Input: part model. Units: mm. Frame: model coordinates. Face numbers are marked on the shaded views. Give positions to 0.01 mm unless a question says otherwise; leave off trailing zeros. Write each loop counter-clockwise with the first axis right and the second up, starting at its lowest first coordinate (ties: lowest second). Pieces come first, ordered by that corner, then holes. Notation, with made-up numbers: (-37.75, 8.5) -> (-14.75, 8.5) arc R24 ccw to (-14.75, 31.5) -> close; hole circle Ø10 at (69.5, 38). An arc over 180 degrees is marked (long way). Return JSON: item names as keys, results as strings. Group by question number.
Item 1: Section A-A, the plane z = 0.5. Return loops of the section in (x, y), then the cut area to 3 significant figures.
Item 2: Pin query (flat end, axial travel): P1, Ø0.5, axis at y = 33.5, z = 2.5, coming from the +X side; P2, Ø0.5, axis at y = 21.5, z = 2.5, coming from the +X side; P3, Ø1.5, axis at x = -6.5, z = 1.5, coming from the -Y side. Return the tip coordinate at first contact, or that it passes through.
Item 3: Section B-B, the plane y = 14. Return loops of the section in (x, z), then the cut area to 3 significant figures.
Item 4: Line query: line 1 (Y direction, x = -11, z = 2.7); line 2 (Y direction, x = -5, z = 2.1); line 3 (Z direction, x = -4, y = 5.5). Output: solid intervals per line, ascending. Write a range as [from, to].
Item 5: Mould query, pull axis Y, two halves, no side actions, for the marked faces 1, 2 and 3. Classes: released by +Y, released by -Y, zero draft, split by the parting line, or undercut.
Item 6: Section D-D, the plane z = 2.55. Count the separate pieces of the cut face and the enclosed holes in it, then the cut area to 3 significant figures.
Item 7: Section C-C, the plane x = -8.5. Return loops of the section in (y, z), then the cut area to 3 significant figures.
Autodesk Inventor part; units mm, degrees
ref_plane "YZ Plane" through (0, 0, 0) normal (1, 0, 0) x (0, 1, 0)
ref_plane "XZ Plane" through (0, 0, 0) normal (0, 1, 0) x (-1, 0, 0)
ref_plane "XY Plane" through (0, 0, 0) normal (0, 0, 1) x (1, 0, 0)
sketch "Sketch1" plane through (0, 0, 0) normal (0, 0, 1) x (1, 0, 0)
  line L0 (0, 0) -> (-30, 0)
  line L1 (-30, 40) -> (0, 40)
  line L2 (-36.1318, 34) -> (13.8682, 34) construction
  circle A0 centre (0, 34) radius 4 construction
  circle A1 centre (-30, 34) radius 4 construction
  line L3 (-30, 30) -> (0, 30) construction
  line L4 (0, 30) -> (4, 34)
  line L5 (4, 34) -> (0, 38)
  line L6 (-30, 30) -> (-26, 34)
  line L7 (-26, 34) -> (-30, 38)
  line L8 (-30, 0) -> (-30, 30)
  line L9 (-30, 38) -> (-30, 40)
  line L10 (0, 40) -> (0, 38)
  line L11 (0, 30) -> (0, 0)
  dimension "d0" = 30
  dimension "d1" = 40
  dimension "d2" = 50
  dimension "d3" = 6
  dimension "d4" = 8
  dimension "d5" = 8
extrude "Extrusion1" add sketch "Sketch1" along normal blind 3
sketch "Sketch2" plane through (0, 0, 3) normal (0, 0, 1) x (1, 0, 0)
  line L0 (-30, 30) -> (-30, 0) construction
  line L1 (-30, 0) -> (0, 0) construction
  line L2 (0, 0) -> (0, 30) construction
  line L3 (-17.303, 36.5) -> (-11.9002, 36.5) construction
  line L4 (-11.9002, 36.5) -> (-11.9002, 30.2072) construction
  line L5 (-11.9002, 30.2072) -> (-17.303, 30.2072) construction
  line L6 (-17.303, 30.2072) -> (-17.303, 36.5) construction
  line L7 (-28.7886, 24) -> (-6.3197, 24)
  line L8 (-6.3197, 24) -> (-6.3197, 26)
  line L9 (-6.3197, 26) -> (-28.7886, 26)
  line L10 (-30, 25) -> (0, 25) construction
  line L11 (-6.3197, 26) -> (-6.3197, 27.5)
  line L12 (-6.3197, 27.5) -> (-1.9896, 25)
  line L13 (-6.3197, 24) -> (-6.3197, 22.5)
  line L14 (-6.3197, 22.5) -> (-1.9896, 25)
  line L15 (-16, 12.2406) -> (-17.5, 12.2406)
  line L16 (-17.5, 12.2406) -> (-15, 7.9105)
  line L17 (-14, 12.2406) -> (-12.5, 12.2406)
  line L18 (-12.5, 12.2406) -> (-15, 7.9105)
  line L19 (-30, 5.5) -> (0, 5.5) construction
  line L20 (-6.9986, 6.5) -> (-1.9986, 6.5)
  line L21 (-1.9986, 6.5) -> (-1.9986, 4.5)
  line L22 (-1.9986, 4.5) -> (-6.9986, 4.5)
  line L23 (-6.9986, 4.5) -> (-6.9986, 6.5)
  line L24 (-6.9986, 6.5) -> (-1.9986, 4.5) construction
  line L25 (-1.9986, 6.5) -> (-6.9986, 4.5) construction
  line L26 (-1.9896, 25) -> (-1.9896, 0) construction
  line L27 (-12.9986, 6.5) -> (-7.9986, 6.5)
  line L28 (-36, 5.5) -> (-6, 5.5) construction
  line L29 (-7.9986, 4.5) -> (-12.9986, 4.5)
  line L30 (-12.9986, 4.5) -> (-12.9986, 6.5)
  line L31 (-7.9986, 6.5) -> (-7.9986, 4.5)
  line L32 (-18.9986, 6.5) -> (-13.9986, 6.5)
  line L33 (-42, 5.5) -> (-12, 5.5) construction
  line L34 (-13.9986, 4.5) -> (-18.9986, 4.5)
  line L35 (-18.9986, 4.5) -> (-18.9986, 5.4478)
  line L36 (-13.9986, 6.5) -> (-13.9986, 4.5)
  line L37 (-24.9986, 6.5) -> (-19.9986, 6.5)
  line L38 (-48, 5.5) -> (-18, 5.5) construction
  line L39 (-19.9986, 4.5) -> (-24.9986, 4.5)
  line L40 (-24.9986, 4.5) -> (-24.9986, 6.5)
  line L41 (-19.9986, 6.5) -> (-19.9986, 4.5)
  line L42 (-24.9986, 6.5) -> (-24.9986, 8)
  line L43 (-24.9986, 8) -> (-29.3287, 5.5)
  line L44 (-24.9986, 4.5) -> (-24.9986, 3)
  line L45 (-24.9986, 3) -> (-29.3287, 5.5)
  line L46 (-28.7886, 26) -> (-28.7886, 24)
  line L47 (-15, 6.5) -> (-15, 7.5)
  line L48 (-15, 7.5) -> (-18.9986, 5.5)
  line L49 (-15, 4.5) -> (-15, 3.5)
  line L50 (-15, 3.5) -> (-18.9986, 5.5)
  line L51 (-15, 6.5) -> (-13.9986, 6.5)
  line L52 (-13.9986, 6.5) -> (-13.9986, 4.5)
  line L53 (-13.9986, 4.5) -> (-15, 4.5)
  line L54 (-15, -0.4455) -> (-15, 27.9265) construction
  line L55 (-16, 12.2406) -> (-16, 17.2406)
  line L56 (-14, 17.2406) -> (-14, 12.2406)
  line L57 (-16, 18.2406) -> (-14, 18.2406)
  line L58 (-14, 18.2406) -> (-14, 23.2406)
  line L59 (-14, 23.2406) -> (-16, 23.2406)
  line L60 (-16, 23.2406) -> (-16, 18.2406)
  line L61 (-16, 17.2406) -> (-14, 17.2406)
  line L62 (0, 40) -> (-30, 40) construction
  line L63 (-11.9643, 30.4) -> (-13.0172, 30.4)
  line L64 (-13.0172, 30.4) -> (-14.9451, 32.8271)
  line L65 (-14.9451, 32.8271) -> (-15.8744, 32.8271)
  line L66 (-15.8744, 32.8271) -> (-15.8744, 30.4)
  line L67 (-15.8744, 30.4) -> (-16.6851, 30.4)
  line L68 (-16.6851, 30.4) -> (-16.6851, 36.5)
  line L69 (-16.6851, 36.5) -> (-15.1132, 36.5)
  spline S0 degree 2 poles (-15.1132, 36.5) (-14.5892, 36.5) (-13.8823, 36.3863) (-13.561, 36.1787) knots 0 0 0 1 2 2 2
  spline S1 degree 2 poles (-13.561, 36.1787) (-13.2397, 35.9711) (-12.8689, 35.3235) (-12.8689, 34.844) knots 0 0 0 1 2 2 2
  spline S2 degree 2 poles (-12.8689, 34.844) (-12.8689, 34.1767) (-13.5511, 33.272) (-14.1344, 33.0545) knots 0 0 0 1 2 2 2
  line L70 (-14.1344, 33.0545) -> (-11.9643, 30.4)
  spline S3 degree 2 poles (-13.7142, 34.7797) (-13.7142, 35.0467) (-13.9021, 35.457) (-14.0998, 35.5904) knots 0 0 0 1 2 2 2
  spline S4 degree 2 poles (-14.0998, 35.5904) (-14.2728, 35.7041) (-14.7325, 35.7981) (-15.0687, 35.7981) knots 0 0 0 1 2 2 2
  line L71 (-15.0687, 35.7981) -> (-15.8744, 35.7981)
  line L72 (-15.8744, 35.7981) -> (-15.8744, 33.5044)
  line L73 (-15.8744, 33.5044) -> (-15.1626, 33.5044)
  spline S5 degree 2 poles (-15.1626, 33.5044) (-14.8116, 33.5044) (-14.253, 33.628) (-14.0602, 33.8207) knots 0 0 0 1 2 2 2
  spline S6 degree 2 poles (-14.0602, 33.8207) (-13.8823, 33.9888) (-13.7142, 34.4634) (-13.7142, 34.7797) knots 0 0 0 1 2 2 2
  point P0 (-30, 24.9574)
  point P1 (-4.4986, 5.5)
  point P2 (-10.4986, 5.5)
  point P3 (-16.4986, 5.5)
  point P4 (-22.4986, 5.5)
  point P5 (-15, 7.9105)
  point P6 (-15, 18.2406)
  point P7 (-15, 40)
  dimension "d18" = 1.5
  dimension "d19" = 5
  dimension "d20" = 1.5
  dimension "d21" = 1.5
  dimension "d22" = 5
  dimension "d23" = 1.5
  dimension "d24" = 5
  dimension "d25" = 2
  dimension "d28" = 6
  dimension "d33" = 1.5
  dimension "d34" = 5
  dimension "d35" = 1.5
  dimension "d38" = 1
  dimension "d39" = 1
  dimension "d40" = 25
  dimension "d41" = 1
  dimension "d42" = 1
  dimension "d43" = 5
  dimension "d44" = 2
  dimension "d45" = 5
  dimension "d47" = 1
  dimension "d48" = 8
  dimension "d49" = 3.5
extrude "Extrusion2" cut sketch "Sketch2" against normal blind 1
properties part number "MS_R[202] text"
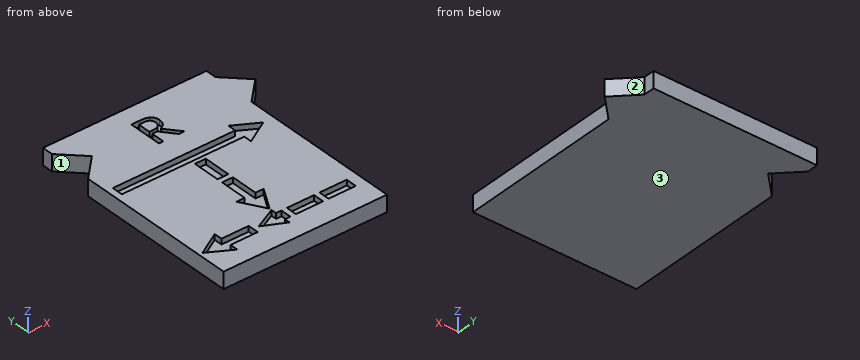
Answer below:
{
 "1": {"outline": "(-30, 0) -> (0, 0) -> (0, 30) -> (4, 34) -> (0, 38) -> (0, 40) -> (-30, 40) -> (-30, 38) -> (-26, 34) -> (-30, 30) -> close", "area": "1,200 mm2"},
 "2": {"P1": "stops at x = 3.75", "P2": "stops at x = 0", "P3": "stops at y = 0"},
 "3": {"outline": "(-30, 0) -> (0, 0) -> (0, 3) -> (-14, 3) -> (-14, 2) -> (-16, 2) -> (-16, 3) -> (-30, 3) -> close", "area": "88.0 mm2"},
 "4": {"line 1": "y = [0, 4.5], [6.5, 24], [26, 40]", "line 2": "y = [0, 4.5], [6.5, 23.26], [26.74, 40]", "line 3": "z = [0, 2]"},
 "5": {"face 1": "undercut", "face 2": "released by +Y", "face 3": "zero draft"},
 "6": {"separate pieces": "2", "enclosed holes": "8", "area": "1,050 mm2"},
 "7": {"outline": "(0, 0) -> (40, 0) -> (40, 3) -> (26, 3) -> (26, 2) -> (24, 2) -> (24, 3) -> (6.5, 3) -> (6.5, 2) -> (4.5, 2) -> (4.5, 3) -> (0, 3) -> close", "area": "116 mm2"}
}
